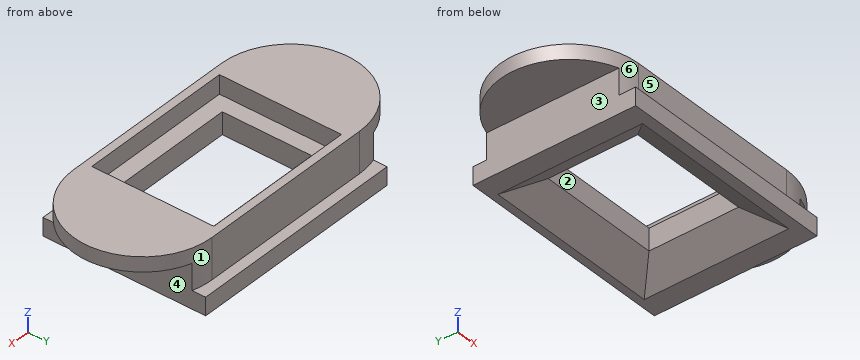
from build123d import *

# Parameters (mm, degrees)
SKETCH_1_W           = 15
SKETCH_1_H           = 11
EXTRUDE_1_DEPTH      = 5
SKETCH_2_W           = 19
SKETCH_2_H           = 15
CUT_EXTRUDE_1_DEPTH  = 2.3
SKETCH_3_OUTSIDE_W   = 49.568
SKETCH_3_OUTSIDE_H   = 27.568
SKETCH_3_OUTSIDE_W_2 = 27
SKETCH_3_OUTSIDE_H_2 = 17
CUT_EXTRUDE_2_DEPTH  = 3.2
SKETCH_4_W           = 27
SKETCH_4_H           = 20
EXTRUDE_2_DEPTH      = 2.2
SKETCH_5_W           = 15
SKETCH_5_H           = 11
CUT_EXTRUDE_3_DEPTH  = 3.2
CUT_EXTRUDE_3_TAPER  = -57


with BuildPart() as part:
    # Эскиз1 → Бобышка-Вытянуть1 (new body)
    with BuildSketch(Plane.XY):
        with BuildLine():
            Line((-11, 8.5), (11, 8.5))
            ThreePointArc((11, 8.5), (19.5, 0), (11, -8.5))
            Line((11, -8.5), (-11, -8.5))
            ThreePointArc((-11, -8.5), (-19.5, 0), (-11, 8.5))
        make_face()
        Rectangle(SKETCH_1_W, SKETCH_1_H, mode=Mode.SUBTRACT)
    extrude(amount=EXTRUDE_1_DEPTH)

    # Эскиз2 → Вырез-Вытянуть1 (cut)
    with BuildSketch(Plane.XY.offset(5)):
        Rectangle(SKETCH_2_W, SKETCH_2_H)
    extrude(amount=-CUT_EXTRUDE_1_DEPTH, mode=Mode.SUBTRACT)

    # Эскиз3 outside → Вырез-Вытянуть2 (cut)
    with BuildSketch(Plane(origin=(0, 0, 0), x_dir=(-1, 0, 0), z_dir=(0, 0, -1))):
        Rectangle(SKETCH_3_OUTSIDE_W, SKETCH_3_OUTSIDE_H)
        Rectangle(SKETCH_3_OUTSIDE_W_2, SKETCH_3_OUTSIDE_H_2, mode=Mode.SUBTRACT)
    extrude(amount=-CUT_EXTRUDE_2_DEPTH, mode=Mode.SUBTRACT)

    # Эскиз4 → Бобышка-Вытянуть2 (add)
    with BuildSketch(Plane(origin=(0, 0, 0), x_dir=(-1, 0, 0), z_dir=(0, 0, -1))):
        with Locations((0, -0.2)):
            Rectangle(SKETCH_4_W, SKETCH_4_H)
    extrude(amount=EXTRUDE_2_DEPTH)

    # Эскиз5 → Вырез-Вытянуть3 (cut, through all)
    with BuildSketch(Plane.XY):
        Rectangle(SKETCH_5_W, SKETCH_5_H)
    extrude(amount=-CUT_EXTRUDE_3_DEPTH, taper=CUT_EXTRUDE_3_TAPER, mode=Mode.SUBTRACT)


solid = part.part
Design review of the part built by this model. Coordinates are the model's own, in mm. Face numbers are marked on the shaded views. A direction names the side the tool comes from. Round coordinates to 2 decimals unless told otherwise and drop trailing zeros. Write each loop counter-clockwise with the first axis right and the second up, starting at its lowest first coordinate (ties: lowest second). Pieces come first, ordered by that corner, then holes. Notation, with made-up numbers: (65.25, 47) -> (113.25, 47) arc R24 cw to (113.25, 62) -> close; hole circle Ø7 at (44.5, -1.5). An arc over 180 degrees is marked (long way). One line per item, written item: value. Start each with the question number.
Q1. The part is to be moulded in two halves that separate along X. For the marked faces 1, 2 and 3, say which applies: pulls with the +X half, pulls with the -X half, needs draft (parallel to the pull), parting line crosses it, or undercut.
Q2. Add section A-A (z = 4). Give the boundary of the cut face in (x, y), then the cut area to 3 significant figures.
Q3. Insertion check: P1, Ø1.5, axis at x = 5.5, z = 3.5, coming from the -Y side; P2, Ø1.5, axis at x = -5, z = 3.5, coming from the +Y side; P3, Ø1.2, axis at y = 2, z = 4, coming from the +X side. Each pin has a flat end and moves straight along its axis. Give the tip position at first contact, or say it passes through.
Q4. To check wall thickness, follow probe 1 along X at (y, z) = (-0.25, 1); probe 2 along Y at (x, z) = (-2, 0.75); probe 3 along Y at (x, z) = (-9, 1.25). State the ranges of each line that lie inside material, in increasing order.
Q5. Tool access review of the marked faces 4, 5 and 6: name each direction out of +Z, -Z, +X, -X, +Y, -Y from which nothing blocks a thin tool from reaching the whole face with its end or side.
Q6. Add section B-B (z = 1.75). Give the boundary of the cut face in (x, y).
Response:
1. face 1: pulls with the +X half
1. face 2: undercut
1. face 3: pulls with the -X half
2. outline: (-11, -8.5) -> (11, -8.5) arc R8.5 ccw to (11, 8.5) -> (-11, 8.5) arc R8.5 ccw to start; hole (-9.5, -7.5) -> (9.5, -7.5) -> (9.5, 7.5) -> (-9.5, 7.5) -> close
2. area: 316 mm^2
3. P1: stops at y = -8.5
3. P2: stops at y = 8.5
3. P3: stops at x = 19.38
4. probe 1: x = -13.5 to -7.5, 7.5 to 13.5
4. probe 2: y = -8.5 to -5.5, 5.5 to 8.5
4. probe 3: y = -8.5 to 8.5
5. face 4: -Z, +X, +Y, -Y
5. face 5: +Z, +X, -X, -Y
5. face 6: +Z, -X
6. outline: (-13.5, -8.12) arc R8.5 ccw to (-11, -8.5) -> (11, -8.5) arc R8.5 ccw to (13.5, -8.12) -> (13.5, 8.12) arc R8.5 ccw to (11, 8.5) -> (-11, 8.5) arc R8.5 ccw to (-13.5, 8.12) -> close; hole (-7.5, -5.5) -> (7.5, -5.5) -> (7.5, 5.5) -> (-7.5, 5.5) -> close
